```python
from build123d import *

# Parameters (mm, degrees)
ESTRUSIONE_ESTRUSIONE1_DEPTH    = 3
PREFORO_DA_MASCHIARE_M4_1_D     = 3.3
PREFORO_DA_MASCHIARE_M4_1_DEPTH = 40.6
PREFORO_DA_MASCHIARE_M4_1_TIP   = 0.991420021


with BuildPart() as part:
    # Schizzo1 → Estrusione-Estrusione1 (new body)
    with BuildSketch(Plane.XY):
        with BuildLine():
            Line((0, 8), (0, 192))
            ThreePointArc((0, 192), (2.343145751, 197.656854249), (8, 200))
            Line((8, 200), (197, 200))
            ThreePointArc((197, 200), (202.656854249, 197.656854249), (205, 192))
            Line((205, 192), (205, 153.313708499))
            ThreePointArc((205, 153.313708499), (204.39103626, 150.25224104), (202.656854249, 147.656854249))
            Line((202.656854249, 147.656854249), (57.343145751, 2.343145751))
            ThreePointArc((57.343145751, 2.343145751), (54.74775896, 0.60896374), (51.686291501, 0))
            Line((51.686291501, 0), (8, 0))
            ThreePointArc((8, 0), (2.343145751, 2.343145751), (0, 8))
        make_face()
    extrude(amount=ESTRUSIONE_ESTRUSIONE1_DEPTH)

    # Preforo da maschiare M4-1
    with Locations(Plane.XY.offset(3)):
        with Locations((15.44269502, 145.7), (15.44269502, 125.7), (15.44269502, 73.7), (15.44269502, 53.7)):
            Hole(PREFORO_DA_MASCHIARE_M4_1_D / 2, depth=PREFORO_DA_MASCHIARE_M4_1_DEPTH)
            with Locations((0, 0, -(PREFORO_DA_MASCHIARE_M4_1_DEPTH + PREFORO_DA_MASCHIARE_M4_1_TIP / 2))):  # 118° drill point
                Cone(0, PREFORO_DA_MASCHIARE_M4_1_D / 2, PREFORO_DA_MASCHIARE_M4_1_TIP, mode=Mode.SUBTRACT)


solid = part.part
```
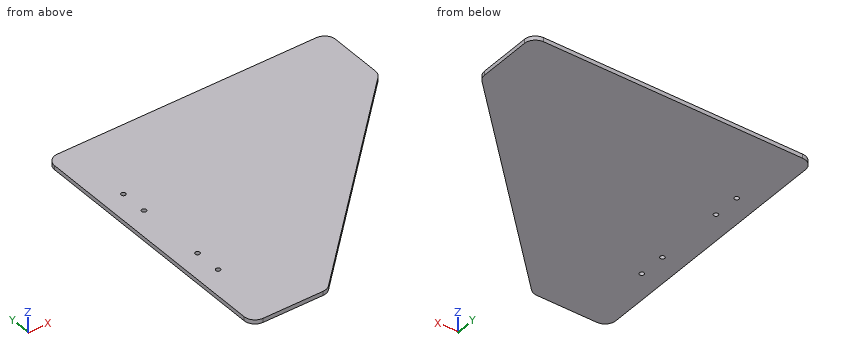
Work out the finished part from the listing and answer in its coordinate system (mm). Round coordinates to 2 decimals unless told otherwise and drop trailing zeros. Loops run counter-clockwise (first coordinate to the right, second up) from the corner with the lowest first, then second, coordinate; pieces in that order, holes last.
(1) The part is cut by section B-B, the plane x = 164. Give the vertices of the cut face in (y, z).
Computed values:
outline: (109, 0) - (200, 0) - (200, 3) - (109, 3) - close
(2) The part is cut by section A-A, the plane z = 0.9. Give the vertices of the cut face in (x, y).
Computed values:
outline: (0, 8) arc R8 ccw to (8, 0) - (51.69, 0) arc R8 ccw to (57.34, 2.34) - (202.66, 147.66) arc R8 ccw to (205, 153.31) - (205, 192) arc R8 ccw to (197, 200) - (8, 200) arc R8 ccw to (0, 192) - close; hole circle Ø3.3 at (15.44, 53.7); hole circle Ø3.3 at (15.44, 73.7); hole circle Ø3.3 at (15.44, 125.7); hole circle Ø3.3 at (15.44, 145.7)
(3) The part is cut by section C-C, the plane y = 34. Give the vertices of the cut face in (x, z).
Computed values:
outline: (0, 0) - (89, 0) - (89, 3) - (0, 3) - close
(4) Find the intervals of material crossed by L1, parallel to X at y = 125.7, z = 1.85; L2, parallel to X at y = 145.7, z = 2.1; L3, parallel to Y at x = 52, z = 0.25, in increasing order.
Computed values:
L1: x = 0 to 13.79, 17.09 to 180.7
L2: x = 0 to 13.79, 17.09 to 200.7
L3: y = 0.01 to 200
(5) This flat-tipped pin is pushed along its axis until it touches: P1, Ø1.5, axis at y = 37.5, z = 1.5, coming from the +X side. Where does it stop, or does it pass through?
Computed values:
P1: stops at x = 93.25
